```python
from build123d import *

# Parameters (mm, degrees)
BOSS_EXTRUDE1_DEPTH        = 60.325
BOSS_EXTRUDE1_DEPTH_BACK   = 60.325
SKETCH3_W                  = 38.1
SKETCH3_H                  = 3.175
F_12_0MM_DOWEL_HOLE1_D     = 12
F_12_0MM_DOWEL_HOLE1_DEPTH = 9.652
F_12_0MM_DOWEL_HOLE1_TIP   = 3.605163714


with BuildPart() as part:
    # Sketch3 → Boss-Extrude1 (new, two sides: drawn at the far end of the back side and taken through both)
    with BuildSketch(Plane.XY.offset(-BOSS_EXTRUDE1_DEPTH_BACK)):
        Rectangle(SKETCH3_W, SKETCH3_H)
    extrude(amount=BOSS_EXTRUDE1_DEPTH + BOSS_EXTRUDE1_DEPTH_BACK)

    # Ø12.0mm Dowel Hole1
    with Locations(Plane(origin=(0, 1.5875, 0), x_dir=(1, 0, 0), z_dir=(0, 1, 0))):
        with Locations((0, 0)):
            Hole(F_12_0MM_DOWEL_HOLE1_D / 2, depth=F_12_0MM_DOWEL_HOLE1_DEPTH)
            with Locations((0, 0, -(F_12_0MM_DOWEL_HOLE1_DEPTH + F_12_0MM_DOWEL_HOLE1_TIP / 2))):  # 118° drill point
                Cone(0, F_12_0MM_DOWEL_HOLE1_D / 2, F_12_0MM_DOWEL_HOLE1_TIP, mode=Mode.SUBTRACT)


solid = part.part
```
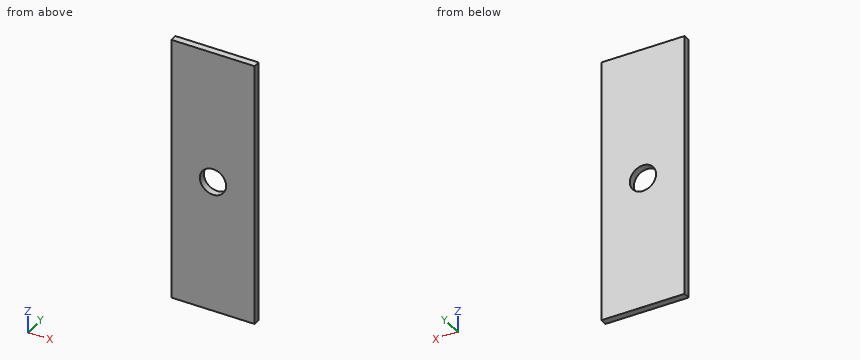
CAD build for the part. Positions are in the model's coordinates, mm. Coordinates: 2 decimals unless noted, no trailing zeros. Write each loop counter-clockwise with the first axis right and the second up, starting at its lowest first coordinate (ties: lowest second). Pieces come first, ordered by that corner, then holes.
(1) Cut at C-C, the plane y = -0.6. List the corners of the cut face in (x, z) (3 decimals).
(2) Drill centre lines: probe 1 along Z at (x, y) = (0, 0.65) (3 decimals); probe 2 along Z at (x, y) = (4.5, 0.25) (3 decimals). Where is each one in solid material? Low to high.
(3) Cut at B-B, the plane x = 0. List the corners of the cut face in (y, z) (1 decimal).
(4) Cut at A-A, the plane z = 0. List the corners of the cut face in (x, y), and give its area (3 significant figures).
Geometry says:
1. outline: (-19.05, -60.325) - (19.05, -60.325) - (19.05, 60.325) - (-19.05, 60.325) - close; hole circle Ø12 at (0, 0)
2. probe 1: z = -60.325 to -6, 6 to 60.325
2. probe 2: z = -60.325 to -3.969, 3.969 to 60.325
3. outline: (-1.6, -60.3) - (1.6, -60.3) - (1.6, -6) - (-1.6, -6) - close; (-1.6, 6) - (1.6, 6) - (1.6, 60.3) - (-1.6, 60.3) - close
4. outline: (-19.05, -1.59) - (-6, -1.59) - (-6, 1.59) - (-19.05, 1.59) - close; (6, -1.59) - (19.05, -1.59) - (19.05, 1.59) - (6, 1.59) - close
4. area: 82.9 mm2
